Study the drawing (mm; zero at the part's minimum x, y, z) and answer. Coordinates: 2 decimals unless noted, no trailing zeros. Loops run counter-clockwise (first coordinate to the right, second up) from the corner with the lowest first, then second, coordinate; pieces in that order, holes last. Notation, with made-up numbers: (41, -4.75) - (53, -4.75) arc R19 cw to (53, 13.25) - close; hole circle Ø2 at (26, -39.75). An arc over 180 degrees is marked (long way). Use one line per item in the form item = value.
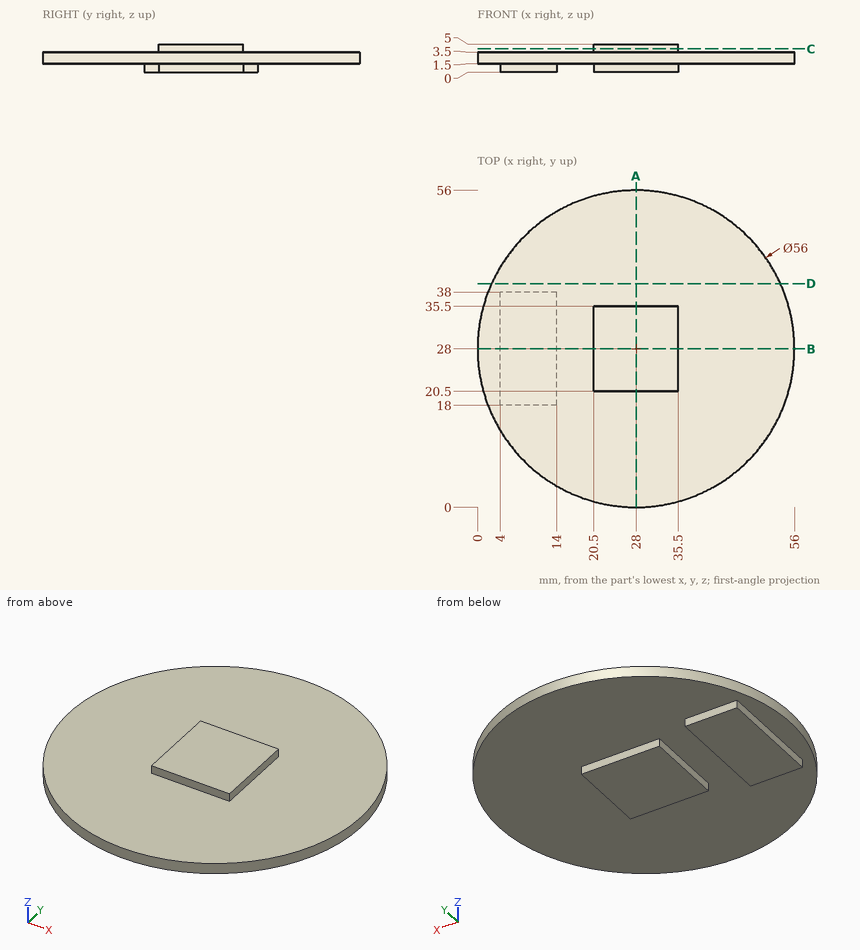
Item 1: The part is cut by section C-C on z = 4.15. Give the vertices of the cut face in (x, y), plus the area to 3 significant figures.
Results below:
outline = (20.5, 20.5) - (35.5, 20.5) - (35.5, 35.5) - (20.5, 35.5) - close
area = 225 mm²
Item 2: The part is cut by section A-A on x = 28. Give the vertices of the cut face in (y, z).
Results below:
outline = (0, 1.5) - (20.5, 1.5) - (20.5, 0) - (35.5, 0) - (35.5, 1.5) - (56, 1.5) - (56, 3.5) - (35.5, 3.5) - (35.5, 5) - (20.5, 5) - (20.5, 3.5) - (0, 3.5) - close
Item 3: Find the intervals of material crossed by L1, parallel to Z at x = 32, y = 48.5; L2, parallel to Y at x = 21.5, z = 1.4, in increasing order.
Results below:
L1 = 1.5 to 3.5
L2 = 20.5 to 35.5
Item 4: Each of these flat-tipped pins is pushed along its axis until it touches: P1, Ø1.6, axis at y = 29.5, z = 4, coming from the -X side; P2, Ø1.6, axis at x = 10, z = 1, coming from the -Y side; P3, Ø1.2, axis at y = 26.5, z = 0.5, coming from the -X side. Where does it stop, or does it pass through?
Results below:
P1 = 0.01
P2 = 6.04
P3 = 4
Item 5: The part is cut by section B-B on y = 28. Give the vertices of the cut face in (x, z).
Results below:
outline = (0, 1.5) - (4, 1.5) - (4, 0) - (14, 0) - (14, 1.5) - (20.5, 1.5) - (20.5, 0) - (35.5, 0) - (35.5, 1.5) - (56, 1.5) - (56, 3.5) - (35.5, 3.5) - (35.5, 5) - (20.5, 5) - (20.5, 3.5) - (0, 3.5) - close
Item 6: The part is cut by section D-D on y = 39.5. Give the vertices of the cut face in (x, z).
Results below:
outline = (2.47, 1.5) - (53.53, 1.5) - (53.53, 3.5) - (2.47, 3.5) - close
